```python
from build123d import *

# Parameters (mm, degrees)
SKETCH1_W           = 150
SKETCH1_H           = 80
BOSS_EXTRUDE1_DEPTH = 5
SKETCH2_W           = 2
SKETCH2_H           = 80
SKETCH2_W_2         = 7
BOSS_EXTRUDE2_DEPTH = 6
BOSS_EXTRUDE3_REACH = 172.356


with BuildPart() as part:
    # Sketch1 → Boss-Extrude1 (new body)
    with BuildSketch(Plane(origin=(0, 0, 0), x_dir=(1, 0, 0), z_dir=(0, 1, 0))):
        with Locations((75, 40)):
            Rectangle(SKETCH1_W, SKETCH1_H)
    extrude(amount=BOSS_EXTRUDE1_DEPTH)

    # Sketch2 → Boss-Extrude2 (add)
    with BuildSketch(Plane(origin=(0, 5, 0), x_dir=(1, 0, 0), z_dir=(0, 1, 0))):
        with Locations((1, 40)):
            Rectangle(SKETCH2_W, SKETCH2_H)
        with Locations((12, 40)):
            Rectangle(SKETCH2_W, SKETCH2_H)
        with Locations((23, 40)):
            Rectangle(SKETCH2_W, SKETCH2_H)
        with Locations((34, 40)):
            Rectangle(SKETCH2_W, SKETCH2_H)
        with Locations((45, 40)):
            Rectangle(SKETCH2_W, SKETCH2_H)
        with Locations((56, 40)):
            Rectangle(SKETCH2_W, SKETCH2_H)
        with Locations((67, 40)):
            Rectangle(SKETCH2_W, SKETCH2_H)
        with Locations((78, 40)):
            Rectangle(SKETCH2_W, SKETCH2_H)
        with Locations((89, 40)):
            Rectangle(SKETCH2_W, SKETCH2_H)
        with Locations((100, 40)):
            Rectangle(SKETCH2_W, SKETCH2_H)
        with Locations((111, 40)):
            Rectangle(SKETCH2_W, SKETCH2_H)
        with Locations((122, 40)):
            Rectangle(SKETCH2_W, SKETCH2_H)
        with Locations((133, 40)):
            Rectangle(SKETCH2_W, SKETCH2_H)
        with Locations((146.5, 40)):
            Rectangle(SKETCH2_W_2, SKETCH2_H)
    extrude(amount=BOSS_EXTRUDE2_DEPTH)

    # Boss-Extrude3: up to this face of the body (flat: up to its plane)
    boss_extrude3_end = Plane(part.part.faces().sort_by_distance((150, 5.5, -40))[0])
    # Sketch3 → Boss-Extrude3 (add, up to the picked face)
    with BuildSketch(Plane.ZY, mode=Mode.PRIVATE) as boss_extrude3_sk1:
        Polygon((0, 0), (0, 5), (5, 0), align=None)
    boss_extrude3_tool1 = split(extrude(boss_extrude3_sk1.sketch, amount=-BOSS_EXTRUDE3_REACH, mode=Mode.PRIVATE), bisect_by=boss_extrude3_end, keep=Keep.BOTH, mode=Mode.PRIVATE)
    add(boss_extrude3_tool1.solids().sort_by(Axis((0, 1.666667, 1.666667), (1, 0, 0)))[0])


solid = part.part
```
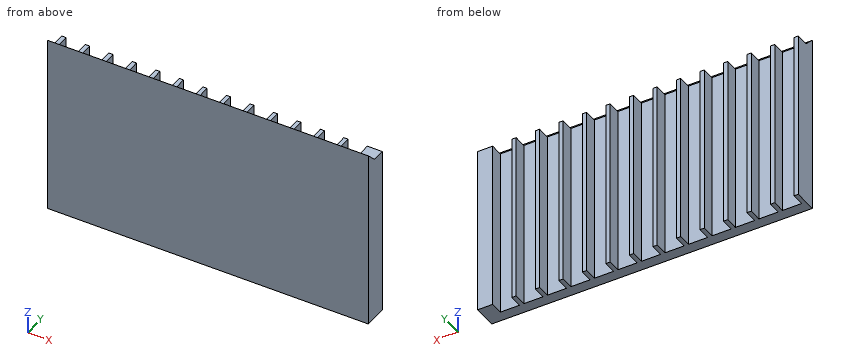
Could you check a few things on this model? Use its own coordinates, in mm. Coordinates: 2 decimals unless noted, no trailing zeros. Write each loop counter-clockwise with the first axis right and the second up, starting at its lowest first coordinate (ties: lowest second). Pieces come first, ordered by that corner, then holes. Notation, with made-up numbers: (46.25, 12) - (62.25, 12) arc R27 cw to (62.25, 32) - close; hole circle Ø3 at (-6, -20). An arc over 180 degrees is marked (long way). Use a Markdown table: item, result.
Q1. Imagine slicing it at A-A (x = 63). List the corners of the cut face in (y, z) for me, and give its area (4 significant figures).
Geometry check:
| item | result |
|---|---|
| outline | (0, -80) - (5, -80) - (5, 0) - (0, 5) - close |
| area | 412.5 mm2 |
Q2. Imagine slicing it at B-B (y = 7). Count the separate pieces of the cut face and the enclosed holes in it, and give its area (3 significant figures).
Geometry check:
| item | result |
|---|---|
| separate pieces | 14 |
| enclosed holes | 0 |
| area | 2,640 mm2 |
Q3. Please list where these lines run through material, in increasing order: L1, parallel to Y at x = 41, z = -26; L2, parallel to Z at x = 34, y = 6.75; L3, parallel to Z at x = 92, y = 1.75.
Geometry check:
| item | result |
|---|---|
| L1 | y = 0 to 5 |
| L2 | z = -80 to 0 |
| L3 | z = -80 to 3.25 |
Q4. I'm going to push flat-ended pins straight in: pin 1 Ø4 at (x, z) = (63.5, -9.5) entering from +Y; pin 2 Ø1.6 at (x, y) = (111, 8.5) entering from +Z. Where does each tip first touch, or does it pass through?
Geometry check:
| item | result |
|---|---|
| pin 1 | stops at y = 5 |
| pin 2 | stops at z = 0 |
